The listing builds one solid part. Answer for the finished solid, in the listing's coordinates (mm). Face numbers are marked on the shaded views. A direction names the side the tool comes from. Give positions to 0.01 mm unless a question says otherwise; leave off trailing zeros. Order: outer loops, then holes, each group sorted by start corner. A loop starts at its lowest first (then second) coordinate and runs counter-clockwise, first axis right, second up.
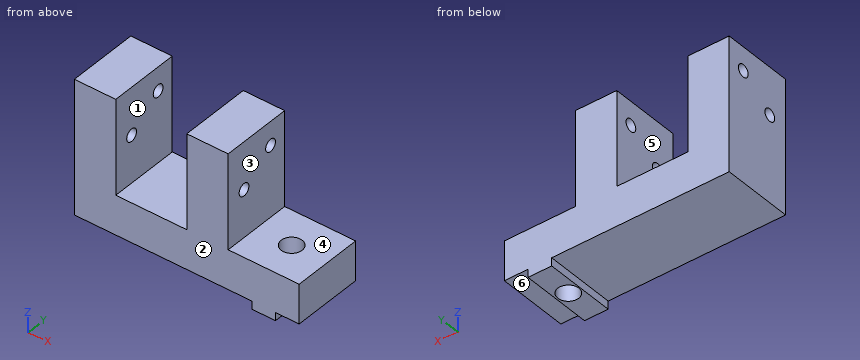
```python
from build123d import *

# Parameters (mm, degrees)
EXTRUDE1_DEPTH         = 9.525
M4X0_7_TAPPED_HOLE1_D  = 3.3
F_10_CLEARANCE_HOLE1_D = 5.6134


with BuildPart() as part:
    # Sketch1 → Extrude1 (new, symmetric)
    with BuildSketch(Plane(origin=(0, 0, 0), x_dir=(1, 0, 0), z_dir=(0, 1, 0))):
        Polygon((47.625, 0), (53.975, 0), (53.975, -2.159), (60.325, -2.159), (60.325, -12.7), (41.275, -12.7), (41.275, -38.1), (30.1625, -38.1), (30.1625, -12.7), (11.1125, -12.7), (11.1125, -38.1), (0, -38.1), (0, -2.159), (47.625, -2.159), align=None)
    extrude(amount=EXTRUDE1_DEPTH, both=True)

    # M4x0.7 Tapped Hole1 (through all)
    with Locations(Plane(origin=(41.275, 0, 0), x_dir=(0, 0, -1), z_dir=(1, 0, 0))):
        with Locations((-31.75, 4.7625), (-25.4, -4.1783)):
            Hole(M4X0_7_TAPPED_HOLE1_D / 2)

    # #10 Clearance Hole1 (through all)
    with Locations(Plane(origin=(0, 0, 0), x_dir=(-1, 0, 0), z_dir=(0, 0, -1))):
        with Locations((-50.7365, 0)):
            Hole(F_10_CLEARANCE_HOLE1_D / 2)


solid = part.part
```
1) Find section B-B (z = 31.75). Write down the section's boundary in (x, y) (1 decimal).
Geometry says:
outline: (0, -9.5) - (11.1, -9.5) - (11.1, 3.1) - (0, 3.1) - close; (0, 6.4) - (11.1, 6.4) - (11.1, 9.5) - (0, 9.5) - close; (30.2, -9.5) - (41.3, -9.5) - (41.3, 3.1) - (30.2, 3.1) - close; (30.2, 6.4) - (41.3, 6.4) - (41.3, 9.5) - (30.2, 9.5) - close
2) Find section D-D (x = 51). Write down the section's boundary in (y, z) (3 decimals), then the cut area to 3 significant figures.
Geometry says:
outline: (-9.525, 0) - (-2.794, 0) - (-2.794, 12.7) - (-9.525, 12.7) - close; (2.794, 0) - (9.525, 0) - (9.525, 12.7) - (2.794, 12.7) - close
area: 171 mm2
3) Given P1, Ø5, axis at y = 7.5, z = 24, coming from the +X side (3 decimals); P2, Ø0.6, axis at y = 1.5, z = 1.5, coming from the -X side (3 decimals); P3, Ø3, axis at x = 51.5, y = 6.5, coming from the +Z side, each flat-ended and moving along its own axis, determine where each tip first touches the part or whether it passes through.
Geometry says:
P1: stops at x = 41.275
P2: stops at x = 47.625
P3: stops at z = 12.7
4) Straight lines are drawn through the part: probe 1 along X at (y, z) = (7, 25.5) (1 decimal); probe 2 along Z at (x, y) = (5, 1); probe 3 along Z at (x, y) = (53, -7.75). For each, find the intervals that lie inside material, in ascending order.
Geometry says:
probe 1: x = 0 to 11.1, 30.2 to 41.3
probe 2: z = 2.16 to 38.1
probe 3: z = 0 to 12.7
5) For a pull along X with two mould halves and no side action, classify the marked faces 1, 2 and 3 as +X half, -X half, draft (parallel to the pull), parting line (faces both ways), or undercut.
Geometry says:
face 1: undercut
face 2: draft
face 3: +X half
6) A tool of negligible diameter and unlimited length cuts with its end or side. For the marked faces 4, 5 and 6, from which of +Z, -Z, +X, -X, +Y, -Y can it reach the whole face along a straight path? Write none if from no direction.
Geometry says:
face 4: +Z, +X, +Y, -Y
face 5: +Z, +Y, -Y
face 6: -Z, +X, +Y, -Y
7) Find section C-C (z = 18.5). Write down the section's boundary in (x, y) (1 decimal), then the cut area to 3 significant figures.
Geometry says:
outline: (0, -9.5) - (11.1, -9.5) - (11.1, 9.5) - (0, 9.5) - close; (30.2, -9.5) - (41.3, -9.5) - (41.3, 9.5) - (30.2, 9.5) - close
area: 423 mm2
